from build123d import *

# Parameters (mm, degrees)
BOSS_EXTRUDE1_DEPTH = 12
SKETCH2_R           = 1.6
CUT_EXTRUDE1_DEPTH  = 21
SKETCH3_R           = 1.6
CUT_EXTRUDE2_DEPTH  = 21


with BuildPart() as part:
    # Sketch1 → Boss-Extrude1 (new body)
    with BuildSketch(Plane.XY):
        Polygon((0, 0), (20, 0), (20, 1), (1, 1), (1, 20), (0, 20), align=None)
    extrude(amount=BOSS_EXTRUDE1_DEPTH)

    # Sketch2 → Cut-Extrude1 (cut, through all)
    with BuildSketch(Plane.XZ):
        with Locations((10, 6)):
            Circle(SKETCH2_R)
    extrude(amount=-CUT_EXTRUDE1_DEPTH, mode=Mode.SUBTRACT)

    # Sketch3 → Cut-Extrude2 (cut, through all)
    with BuildSketch(Plane.ZY):
        with Locations((6, 10)):
            Circle(SKETCH3_R)
    extrude(amount=-CUT_EXTRUDE2_DEPTH, mode=Mode.SUBTRACT)


solid = part.part
Build history of the part. All positions in model axes, mm. A direction names the side the tool comes from. Round coordinates to 2 decimals unless told otherwise and drop trailing zeros. Write each loop counter-clockwise with the first axis right and the second up, starting at its lowest first coordinate (ties: lowest second). Pieces come first, ordered by that corner, then holes. Notation, with made-up numbers: M -29.75,-27 L -3.75,-27 A12 ccw -3.75,-14 Z; hole C 7.5,4 d11. An arc over 180 degrees is marked long. Use CSV: the item, a comma, the result in double quotes.
1. Saw through at A-A (y = 10). Give the cut face in (x, z), plus the area to 3 significant figures.
Reply:
outline,"M 0,0 L 1,0 L 1,4.4 L 0,4.4 Z; M 0,7.6 L 1,7.6 L 1,12 L 0,12 Z"
area,"8.80 mm²"
2. Wall check: probe 1 along Y at (x, z) = (0.5, 6); probe 2 along X at (y, z) = (6.75, 10.75); probe 3 along Z at (x, y) = (10, 0.8). Give the ranges that are in metal, low to high. Write a range as from..to.
Reply:
probe 1,"y = 0..8.4, 11.6..20"
probe 2,"x = 0..1"
probe 3,"z = 0..4.4, 7.6..12"
3. Saw through at B-B (z = 6). Give the cut face in (x, y), plus the area to 3 significant figures.
Reply:
outline,"M 0,0 L 8.4,0 L 8.4,1 L 1,1 L 1,8.4 L 0,8.4 Z; M 0,11.6 L 1,11.6 L 1,20 L 0,20 Z; M 11.6,0 L 20,0 L 20,1 L 11.6,1 Z"
area,"32.6 mm²"
4. Saw through at C-C (x = 15.25). Give the cut face in (y, z).
Reply:
outline,"M 0,0 L 1,0 L 1,12 L 0,12 Z"
5. Tool access for faces 4 (the face through (13, 1, 6)), 5 (the face through (0.5, 20, 5.9)): list every direction of +Z, -Z, +X, -X, +Y, -Y with a clear straight run to the whole face (end or side of a thin tool).
Reply:
face 4,"+Z, -Z, +X, +Y"
face 5,"+Z, -Z, +X, -X, +Y"
6. Saw through at D-D (z = 3.75). Give the cut face in (x, y), plus the area to 3 significant figures.
Reply:
outline,"M 0,0 L 20,0 L 20,1 L 1,1 L 1,20 L 0,20 Z"
area,"39.0 mm²"
7. Flat gauge pins, fed straight in: pin 1 (5 mm diameter, centred on x = 13.5, z = 1, fed in from -Y); pin 2 (3.5 mm diameter, centred on y = 10, z = 6.5, fed in from +X); pin 3 (1 mm diameter, centred on x = 5.5, z = 8, fed in from +Y). Where does each tip first touch, or does it go through?
Reply:
pin 1,"stops at y = 0"
pin 2,"stops at x = 1"
pin 3,"stops at y = 1"
8. Two-plate mould, pull along Z, no slides. Class faces 1 (the face through (1, 8, 6)), 2 (the face through (8.4, 0.49, 6.07)), 3 (the face through (0.3, 5.6, 0)): +Z half, -Z half, draft (parallel to the pull), parting line (faces both ways), or undercut.
Reply:
face 1,"draft"
face 2,"undercut"
face 3,"-Z half"
